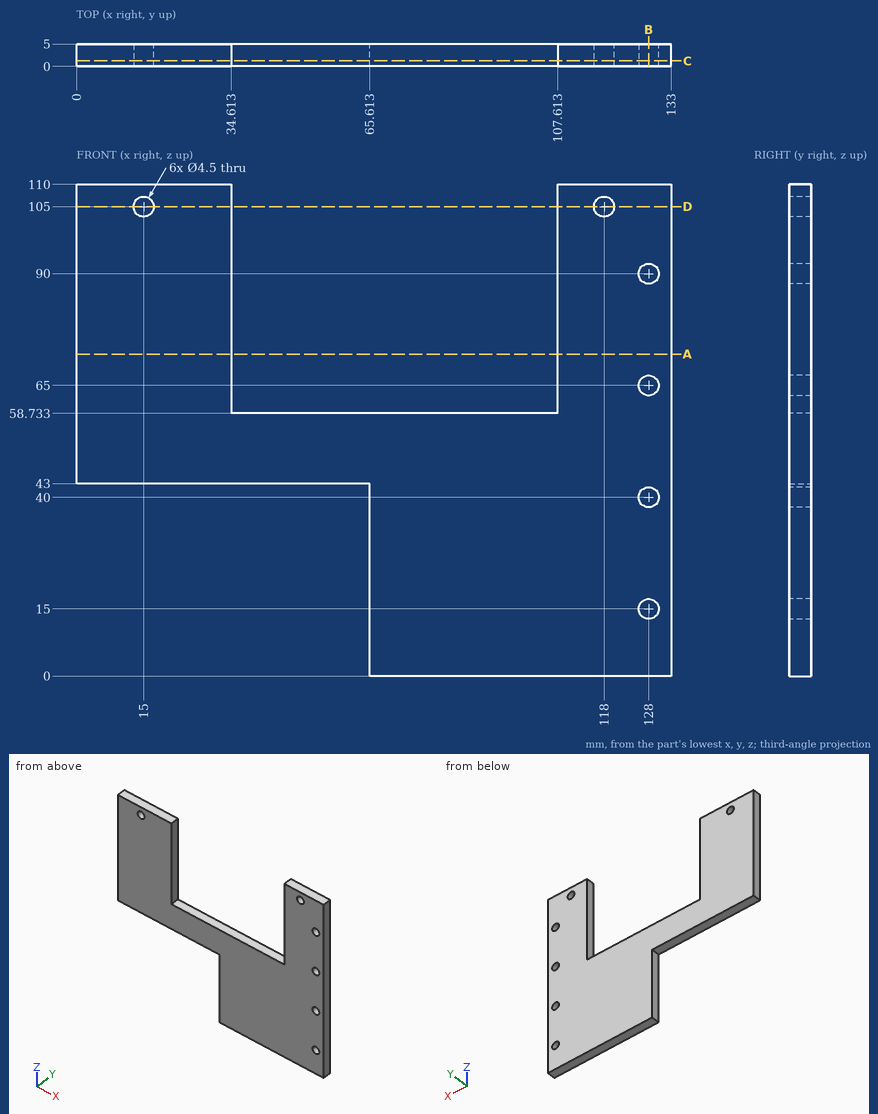
Check sheet for the drawn part. Datum: minimum x, y, z corner. Units: mm. Give positions to 0.01 mm unless a question says otherwise; leave off trailing zeros. Write each loop counter-clockwise with the first axis right and the second up, starting at its lowest first coordinate (ties: lowest second). Pieces come first, ordered by that corner, then holes. Notation, with made-up numbers: (-33.5, 64) -> (6.5, 64) arc R30 ccw to (6.5, 93) -> close; hole circle Ø8 at (-36, 38.5). An arc over 180 degrees is marked (long way). Use one line per item in the form item = value. Start each with the question number.
1. Section check C-C (y = 1.2). Record the cut outline in (x, z), and give its area (3 significant figures).
2. Go/stop test with flat-tipped pins: P1, Ø7, axis at x = 118, z = 105, coming from the +Y side; P2, Ø4, axis at x = 15, z = 105, coming from the -Y side; P3, Ø2.5, axis at x = 17, y = 2.5, coming from the -Z side. Record where each tip stops, or that it passes through.
3. Section check D-D (z = 105). Record the cut outline in (x, y), and give its area (3 significant figures).
4. Thickness scan on line 1 along Z through (x, y) = (128, 3.5); line 2 along X through (y, z) = (3.4, 105); line 3 along X through (y, z) = (1, 65). Record the ranges inside material, lowest first. Write a range as from..to.
5. Section check B-B (x = 128). Record the cut outline in (y, z).
6. Section check A-A (z = 72). Record the cut outline in (x, y).
Conclusion:
q1.outline = (0, 43) -> (65.61, 43) -> (65.61, 0) -> (133, 0) -> (133, 110) -> (107.61, 110) -> (107.61, 58.73) -> (34.61, 58.73) -> (34.61, 110) -> (0, 110) -> close; hole circle Ø4.5 at (15, 105); hole circle Ø4.5 at (118, 105); hole circle Ø4.5 at (128, 15); hole circle Ø4.5 at (128, 40); hole circle Ø4.5 at (128, 65); hole circle Ø4.5 at (128, 90)
q1.area = 7,970 mm²
q2.P1 = 5
q2.P2 = through
q2.P3 = 43
q3.outline = (0, 0) -> (12.75, 0) -> (12.75, 5) -> (0, 5) -> close; (17.25, 0) -> (34.61, 0) -> (34.61, 5) -> (17.25, 5) -> close; (107.61, 0) -> (115.75, 0) -> (115.75, 5) -> (107.61, 5) -> close; (120.25, 0) -> (133, 0) -> (133, 5) -> (120.25, 5) -> close
q3.area = 255 mm²
q4.line_1 = 0..12.75, 17.25..37.75, 42.25..62.75, 67.25..87.75, 92.25..110
q4.line_2 = 0..12.75, 17.25..34.61, 107.61..115.75, 120.25..133
q4.line_3 = 0..34.61, 107.61..125.75, 130.25..133
q5.outline = (0, 0) -> (5, 0) -> (5, 12.75) -> (0, 12.75) -> close; (0, 17.25) -> (5, 17.25) -> (5, 37.75) -> (0, 37.75) -> close; (0, 42.25) -> (5, 42.25) -> (5, 62.75) -> (0, 62.75) -> close; (0, 67.25) -> (5, 67.25) -> (5, 87.75) -> (0, 87.75) -> close; (0, 92.25) -> (5, 92.25) -> (5, 110) -> (0, 110) -> close
q6.outline = (0, 0) -> (34.61, 0) -> (34.61, 5) -> (0, 5) -> close; (107.61, 0) -> (133, 0) -> (133, 5) -> (107.61, 5) -> close
